Model file for the job. Use its own axes, mm. Give positions to 0.01 mm unless a question says otherwise; leave off trailing zeros. Loops run counter-clockwise (first coordinate to the right, second up) from the corner with the lowest first, then second, coordinate; pieces in that order, holes last. Notation, with made-up numbers: (88.5, 16) - (133.5, 16) arc R36 ccw to (133.5, 54) - close; hole circle Ø5 at (-33.5, 40). An arc over 180 degrees is marked (long way). Answer as CSV lines item,"result". Start each with the question number.
Item 1: Saw through at A-A on x = 0. Give the cut face in (y, z), plus the area to 3 significant figures.
Item 2: Saw through at B-B on y = 0. Give the cut face in (x, z).
Item 3: Saw through at C-C on z = -2.5. Give the cut face in (x, y).
Item 4: Drill centre lines: L1, parallel to Y at x = 0, z = 2.5; L2, parallel to Y at x = -1.1, z = -5.5; L3, parallel to X at y = -0.3, z = 1. Where is each one in solid material? Low to high. Write a range as from..to.
Item 5: Pin check, flat tip, straight feed: pin 1 (1 mm diameter, centred on y = 1, z = 4, fed in from +X). Stop position of the tip, or through.
from build123d import *

# Parameters (mm, degrees)
EXTRUDE1_DEPTH = 7.14375


with BuildPart() as part:
    # Sketch1 → Extrude1 (new body, symmetric)
    with BuildSketch(Plane.XY):
        with BuildLine():
            Line((-1.238198788, 0.218327854), (-0.687888215, 0.121293252))
            ThreePointArc((-0.687888215, 0.121293252), (0.6985, 0), (-0.687888215, -0.121293252))
            Line((-0.687888215, -0.121293252), (-1.238198788, -0.218327854))
            ThreePointArc((-1.238198788, -0.218327854), (1.2573, 0), (-1.238198788, 0.218327854))
        make_face()
    extrude(amount=EXTRUDE1_DEPTH, both=True)

    # Sketch2 → Cut-Revolve1 (revolve, cut)
    with BuildSketch(Plane(origin=(0, 0, 0), x_dir=(0, 0, -1), z_dir=(1, 0, 0))):
        Polygon((7.14375, 1.2573), (7.14375, 1.1557), (6.17855, 1.2573), align=None)
        Polygon((-6.17855, 1.2573), (-7.14375, 1.2573), (-7.14375, 1.1557), align=None)
    revolve(axis=Axis((0, 0, -7.14375), (0, 0, 1)), mode=Mode.SUBTRACT)


solid = part.part
Responses:
1,outline,"(-1.26, -6.18) - (-1.16, -7.14) - (-0.7, -7.14) - (-0.7, 7.14) - (-1.16, 7.14) - (-1.26, 6.18) - close; (0.7, -7.14) - (1.16, -7.14) - (1.26, -6.18) - (1.26, 6.18) - (1.16, 7.14) - (0.7, 7.14) - close"
1,area,"15.8 mm2"
2,outline,"(0.7, -7.14) - (1.16, -7.14) - (1.26, -6.18) - (1.26, 6.18) - (1.16, 7.14) - (0.7, 7.14) - close"
3,outline,"(-1.24, -0.22) arc R1.26 ccw (long way) to (-1.24, 0.22) - (-0.69, 0.12) arc R0.7 cw (long way) to (-0.69, -0.12) - close"
4,L1,"-1.26..-0.7, 0.7..1.26"
4,L2,"-0.61..-0.19, 0.19..0.61"
4,L3,"-1.22..-0.63, 0.63..1.22"
5,pin 1,"x = 1.15"
